Design review of the part built by this model. Coordinates are the model's own, in mm. Coordinates: 2 decimals unless noted, no trailing zeros. Write each loop counter-clockwise with the first axis right and the second up, starting at its lowest first coordinate (ties: lowest second). Pieces come first, ordered by that corner, then holes. Notation, with made-up numbers: (48, 11) -> (104, 11) arc R22 ccw to (104, 22) -> close; hole circle Ø1 at (18, 68.25). An arc over 180 degrees is marked (long way). Return JSON: item names as keys, results as strings. Group by question number.
from build123d import *

# Parameters (mm, degrees)
F1_DEPTH = 3


with BuildPart() as f1:
    # F0 (on Front) → F1 (new body)
    with BuildSketch(Plane.XZ):
        with BuildLine():
            Line((2, 0), (6, 0))
            ThreePointArc((6, 0), (0, 6), (-6, 0))
            Line((-6, 0), (-2, 0))
            ThreePointArc((-2, 0), (0, 2), (2, 0))
        make_face()
        with BuildLine():
            Line((6, -50), (6, 0))
            ThreePointArc((6, 0), (0, -6), (-6, 0))
            Line((-6, 0), (-6, -50))
            ThreePointArc((-6, -50), (0, -44), (6, -50))
        make_face()
        with BuildLine():
            ThreePointArc((-6, 0), (0, -6), (6, 0))
            Line((6, 0), (2, 0))
            ThreePointArc((2, 0), (0, -2), (-2, 0))
            Line((-2, 0), (-6, 0))
        make_face()
        with BuildLine():
            Line((2, -50), (6, -50))
            ThreePointArc((6, -50), (0, -44), (-6, -50))
            Line((-6, -50), (-2, -50))
            ThreePointArc((-2, -50), (0, -48), (2, -50))
        make_face()
        with BuildLine():
            ThreePointArc((-6, -50), (0, -56), (6, -50))
            Line((6, -50), (2, -50))
            ThreePointArc((2, -50), (0, -52), (-2, -50))
            Line((-2, -50), (-6, -50))
        make_face()
    extrude(amount=F1_DEPTH)


solid = f1.part
Q1. The part is to be moulded in two halves that separate along X. For faces 1 (the cylindrical face through (0, -1, 6)), 2 (the flat face through (0, 0, -25)), 3 (the cylindrical face through (0, -1, 2)), say which applies: +X half, -X half, draft (parallel to the pull), parting line (faces both ways), or undercut.
Q2. We need section A-A on x = 0. Write out the cut boundary in (y, z).
Q3. Wall thickness on L1, parallel to Z at x = 0, y = -1.45; L2, parallel to X at y = -2.4, z = -50; L3, parallel to Z at x = -1.5, y = -1.4: over which ranges is each line inside the solid? List them lowest first.
Q4. We need section B-B on y = -0.5. Write out the cut boundary in (x, z), plus the area to 3 significant figures.
Q5. For P1, Ø4.5, axis at x = 0, z = 0, coming from the -Y side; P2, Ø3, axis at x = 0, z = -50, coming from the +Y side, all flat-tipped, find the tip position at first contact; note any pin that passes through.
Findings below:
{
 "1": {"face 1": "parting line", "face 2": "draft", "face 3": "undercut"},
 "2": {"outline": "(-3, -56) -> (0, -56) -> (0, -52) -> (-3, -52) -> close; (-3, -48) -> (0, -48) -> (0, -2) -> (-3, -2) -> close; (-3, 2) -> (0, 2) -> (0, 6) -> (-3, 6) -> close"},
 "3": {"L1": "z = -56 to -52, -48 to -2, 2 to 6", "L2": "x = -6 to -2, 2 to 6", "L3": "z = -55.81 to -51.32, -48.68 to -1.32, 1.32 to 5.81"},
 "4": {"outline": "(-6, -50) arc R6 ccw to (6, -50) -> (6, 0) arc R6 ccw to (-6, 0) -> close; hole circle Ø4 at (0, -50); hole circle Ø4 at (0, 0)", "area": "688 mm^2"},
 "5": {"P1": "stops at y = -3", "P2": "passes through"}
}
